from build123d import *

# Parameters (mm, degrees)
F0_W      = 8.75
F0_H      = 8.75
F1_DEPTH  = 7.5
F2_T      = -1.5
F4_DEPTH  = 7.5
F6_DEPTH  = 2.9
F7_R      = 3.25
F8_DEPTH  = 32.25
F9_R      = 3.25
F10_DEPTH = 32.25


with BuildPart() as f1:
    # F0 (on Top) → F1 (new body)
    with BuildSketch(Plane.XY):
        Polygon((25, 0), (25, 8.75), (8.75, 8.75), (0, 8.75), (0, 0), align=None)
        Polygon((25, -8.75), (25, 0), (0, 0), (0, -25), (8.75, -25), (8.75, -8.75), align=None)
        with Locations((-4.375, 4.375)):
            Rectangle(F0_W, F0_H)
        Polygon((0, -25), (0, 0), (-8.75, 0), (-8.75, -8.75), (-8.75, -25), align=None)
    extrude(amount=F1_DEPTH)

    # F2
    f2_openings = [f1.faces().sort_by_distance(p)[0] for p in [
        (5.484375, -5.484375, 7.5),
    ]]
    offset(amount=F2_T, openings=f2_openings, kind=Kind.INTERSECTION)

    # F3 (on face) → F4 (join, through all)
    with BuildSketch(Plane.XY.offset(7.5)):
        Polygon((-4.4215728753, 7.25), (-7.25, 7.25), (-7.25, 4.4215728753), align=None)
        Polygon((11.5784271247, -8.75), (8.75, -8.75), (8.75, -11.5784271247), align=None)
        Polygon((23.5, 7.25), (20.6715728753, 7.25), (23.5, 4.4215728753), align=None)
        Polygon((-4.4215728753, -23.5), (-7.25, -20.6715728753), (-7.25, -23.5), align=None)
    extrude(amount=-F4_DEPTH)

    # F5 (on face) → F6 (join)
    with BuildSketch(Plane.XY.offset(7.5)):
        with BuildLine():
            ThreePointArc((-6.4014718626, 6.4014718626), (-6.2497309366, 6.6285682068), (-6.1964466094, 6.8964466094))
            ThreePointArc((-6.1964466094, 6.8964466094), (-7.5431622822, 7.1643250121), (-6.4014718626, 6.4014718626))
        make_face()
        with BuildLine():
            ThreePointArc((22.6514718626, 6.4014718626), (23.4143250121, 6.2497309366), (23.8464466094, 6.8964466094))
            ThreePointArc((23.8464466094, 6.8964466094), (22.8785682068, 7.5431622822), (22.6514718626, 6.4014718626))
        make_face()
        with BuildLine():
            ThreePointArc((9.5985281374, -9.5985281374), (9.7502690634, -9.3714317932), (9.8035533906, -9.1035533906))
            ThreePointArc((9.8035533906, -9.1035533906), (8.4568377178, -8.8356749879), (9.5985281374, -9.5985281374))
        make_face()
        with BuildLine():
            ThreePointArc((-6.4014718626, -22.6514718626), (-7.5431622822, -23.4143250121), (-6.1964466094, -23.1464466094))
            ThreePointArc((-6.1964466094, -23.1464466094), (-6.2497309366, -22.8785682068), (-6.4014718626, -22.6514718626))
        make_face()
    extrude(amount=F6_DEPTH)

    # F7 (on face) → F8 (cut, through all)
    with BuildSketch(Plane.XZ.offset(25)):
        with Locations((0, 7.5)):
            Circle(F7_R)
    extrude(amount=-F8_DEPTH, mode=Mode.SUBTRACT)

    # F9 (on face) → F10 (cut, through all)
    with BuildSketch(Plane.YZ.offset(25)):
        with Locations((0, 7.5)):
            Circle(F9_R)
    extrude(amount=-F10_DEPTH, mode=Mode.SUBTRACT)


solid = f1.part
The model under review builds one solid part; all positions refer to its coordinate system, in mm. A direction names the side the tool comes from. Give positions to 0.01 mm unless a question says otherwise; leave off trailing zeros. Order: outer loops, then holes, each group sorted by start corner. A loop starts at its lowest first (then second) coordinate and runs counter-clockwise, first axis right, second up. Notation, with made-up numbers: (76.5, 53) -> (103.5, 53) arc R29 cw to (103.5, 74) -> close; hole circle Ø7 at (-1, 44.25). An arc over 180 degrees is marked (long way). Write item = value, one per line. Start each with the question number.
(1) For L1, parallel to Y at x = 16.5, z = 1.75; L2, parallel to Y at x = 7, z = 4.25, list the stretches that pass through material, from the lowest coordinate up. Write a range as from..to.
(2) Take a section at C-C (x = 0). Write out the cut boundary in (y, z), plus the area to 4 significant figures.
(3) Tool access review of faces 1 (the cylindrical face through (24.26, -0.07, 4.25)), 2 (the flat face through (18, -8.75, 4)), 3 (the flat face through (7.25, -15, 4)), 4 (the cylindrical face through (-0.07, -24.26, 4.25)): name each direction out of +Z, -Z, +X, -X, +Y, -Y from which nothing blocks a thin tool from reaching the whole face with its end or side.
(4) Take a section at A-A (z = 8.5). Write out the cut boundary in (x, y), plus the area to 3 significant figures.
(5) Take a section at B-B (z = 6.75). Write out the cut boundary in (x, y), plus the area to 3 significant figures.
(6) Take a section at D-D (y = 0). Write out the cut boundary in (x, z), plus the area to 4 significant figures.
(7) Draft analysis for pull direction X (two halves, no side actions). For faces 5 (the flat face through (4, -4, 0)), 6 (the flat face through (25, 0, 4)), 7 (the flat face through (8, 7.25, 4)), state which applies: +X half, -X half, draft (parallel to the pull), parting line (faces both ways), or undercut.
(8) For pin 1 Ø8 at (x, y) = (13, 3.5) entering from +Z; pin 2 Ø4 at (x, y) = (-3, -14.5) entering from +Z; pin 3 Ø6 at (x, z) = (16.5, 3) entering from -Y, all flat-tipped, find the tip position at first contact; note any pin that passes through.
Returned:
q1.L1 = -8.75..-7.25, 7.25..8.75
q1.L2 = -25..-23.5, 7.25..8.75
q2.outline = (-25, 0) -> (8.75, 0) -> (8.75, 7.5) -> (7.25, 7.5) -> (7.25, 1.5) -> (-23.5, 1.5) -> (-23.5, 4.25) -> (-25, 4.25) -> close
q2.area = 63.75 mm²
q3.face_1 = +Z, +X
q3.face_2 = +Z, -Z, +X, -Y
q3.face_3 = +Z
q3.face_4 = +Z, -Y
q4.outline = circle Ø1.4 at (-6.9, -23.15); circle Ø1.4 at (-6.9, 6.9); circle Ø1.4 at (9.1, -9.1); circle Ø1.4 at (23.15, 6.9)
q4.area = 6.16 mm²
q5.outline = (-8.75, -25) -> (-3.16, -25) -> (-3.16, -23.5) -> (-4.42, -23.5) -> (-7.25, -20.67) -> (-7.25, 4.42) -> (-4.42, 7.25) -> (20.67, 7.25) -> (23.5, 4.42) -> (23.5, 3.16) -> (25, 3.16) -> (25, 8.75) -> (-8.75, 8.75) -> close; (3.16, -25) -> (8.75, -25) -> (8.75, -11.58) -> (11.58, -8.75) -> (25, -8.75) -> (25, -3.16) -> (23.5, -3.16) -> (23.5, -7.25) -> (7.25, -7.25) -> (7.25, -23.5) -> (3.16, -23.5) -> close
q5.area = 191 mm²
q6.outline = (-8.75, 0) -> (25, 0) -> (25, 4.25) -> (23.5, 4.25) -> (23.5, 1.5) -> (-7.25, 1.5) -> (-7.25, 7.5) -> (-8.75, 7.5) -> close
q6.area = 63.75 mm²
q7.face_5 = draft
q7.face_6 = +X half
q7.face_7 = undercut
q8.pin_1 = 7.5
q8.pin_2 = 1.5
q8.pin_3 = -8.75
